Input: dimensioned drawing with shaded views. Units: mm. Origin: part minimum x, y, z. Give positions to 0.01 mm unless a question says otherwise; leave off trailing zeros. Order: outer loops, then holes, each group sorted by start corner. A loop starts at its lowest first (then second) coordinate and runs counter-clockwise, first axis right, second up. Notation, with made-up numbers: (20, 12.25) - (35, 12.25) arc R29 cw to (35, 35.25) - close; hole circle Ø9 at (35, 37.5). An arc over 180 degrees is marked (long way). Answer as CSV lines item,"result".
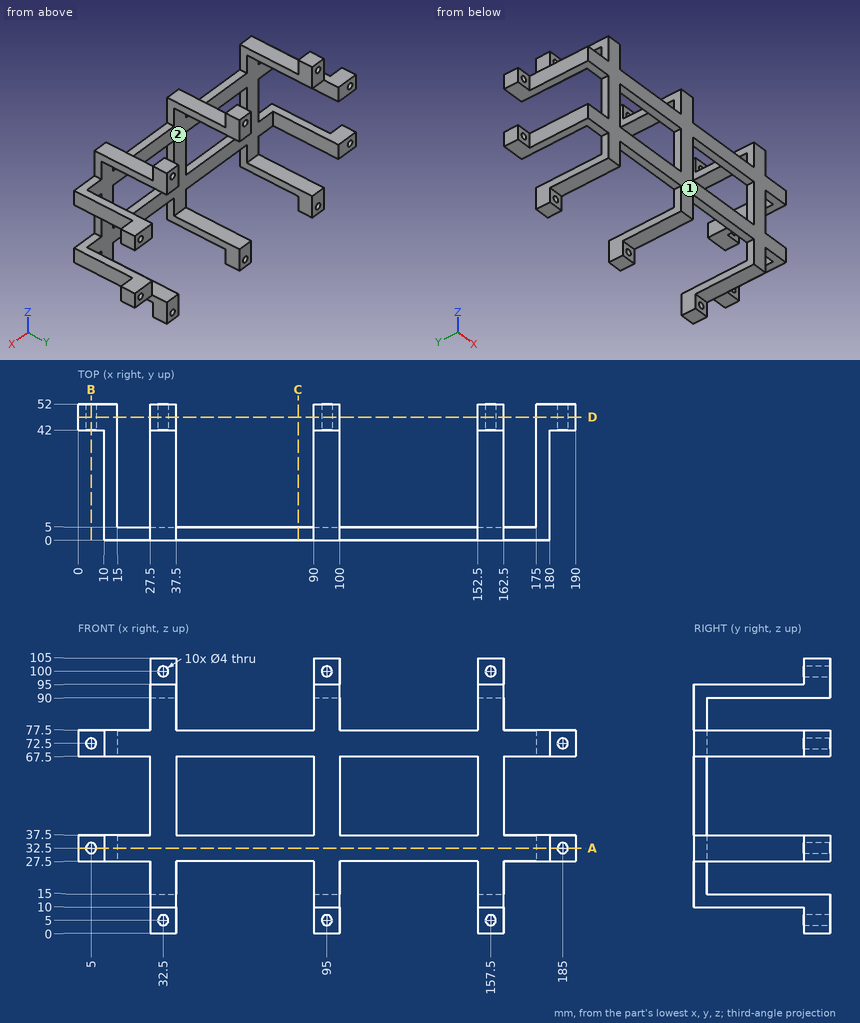
(1) Cut plane C-C (x = 84). Return loops of the section in (y, z), then the cut area to 3 significant figures.
Completed:
outline,"(0, 27.5) - (5, 27.5) - (5, 37.5) - (0, 37.5) - close; (0, 67.5) - (5, 67.5) - (5, 77.5) - (0, 77.5) - close"
area,"100 mm²"
(2) Cut plane B-B (x = 5). Return loops of the section in (y, z).
Completed:
outline,"(42, 27.5) - (52, 27.5) - (52, 30.5) - (42, 30.5) - close; (42, 34.5) - (52, 34.5) - (52, 37.5) - (42, 37.5) - close; (42, 67.5) - (52, 67.5) - (52, 70.5) - (42, 70.5) - close; (42, 74.5) - (52, 74.5) - (52, 77.5) - (42, 77.5) - close"
(3) Cut plane A-A (z = 32.5). Return loops of the section in (x, y), then the cut area to 3 significant figures.
Completed:
outline,"(0, 42) - (3, 42) - (3, 52) - (0, 52) - close; (7, 42) - (10, 42) - (10, 0) - (180, 0) - (180, 42) - (183, 42) - (183, 52) - (175, 52) - (175, 5) - (15, 5) - (15, 52) - (7, 52) - close; (187, 42) - (190, 42) - (190, 52) - (187, 52) - close"
area,"1,440 mm²"
(4) Ray query, line 1 (X direction, y = 44.75, z = 32.5); line 2 (X direction, y = 49.25, z = 5); line 3 (Z direction, x = 185, y = 46). Return the intervals inside material, ascending. Write a range as from..to.
Completed:
line 1,"0..3, 7..15, 175..183, 187..190"
line 2,"27.5..30.5, 34.5..37.5, 90..93, 97..100, 152.5..155.5, 159.5..162.5"
line 3,"27.5..30.5, 34.5..37.5, 67.5..70.5, 74.5..77.5"
(5) Cut plane D-D (y = 47). Give the number of separate pieces and of enclosed holes in the cut face, then the cut area to 3 significant figures.
Completed:
separate pieces,"10"
enclosed holes,"10"
area,"1,370 mm²"
(6) Mould query, pull axis X, two halves, no side actions, for the marked faces 1 and 2. Classes: released by +X, released by -X, zero draft, split by the parting line, or undercut.
Completed:
face 1,"zero draft"
face 2,"undercut"
(7) Contact query for flat-ended pins moving along their axis: pin 1 (5.5 mm diameter, centred on x = 125, y = 3, fed in from -Z); pin 2 (3 mm diameter, centred on x = 156, y = 19.5, fed in from +Z); pin 3 (4 mm diameter, centred on x = 132, z = 36.5, fed in from +Y). Output: stop coordinate, or through.
Completed:
pin 1,"z = 27.5"
pin 2,"z = 95"
pin 3,"y = 5"
